from build123d import *

# Parameters (mm, degrees)
F0_R      = 50
F1_DEPTH  = 60
F3_DEPTH  = 60.001
F4_W      = 50
F4_H      = 50
F5_DEPTH  = 140
F6_W      = 30
F6_H      = 59.9
F7_DEPTH  = 49.99
F13_DEPTH = 50.0010001
F15_DEPTH = 50.0010001


with BuildPart() as f1:
    # F0 (on Top) → F1 (new body)
    with BuildSketch(Plane.XY):
        Circle(F0_R)
    extrude(amount=F1_DEPTH)

    # F2 (on face) → F3 (cut, through all)
    with BuildSketch(Plane.XY.offset(60)):
        with BuildLine():
            Line((0, -50), (0, 0))
            Line((0, 0), (-50, 0))
            ThreePointArc((-50, 0), (-35.3553390593, -35.3553390593), (0, -50))
        make_face()
    extrude(amount=-F3_DEPTH, mode=Mode.SUBTRACT)

    # F4 (on Top) → F5 (join)
    with BuildSketch(Plane.XY):
        with Locations((-25, -25)):
            Rectangle(F4_W, F4_H)
    extrude(amount=F5_DEPTH)

    # F6 (on face) → F7 (cut)
    with BuildSketch(Plane(origin=(-50, 0, 0), x_dir=(0, -1, 0), z_dir=(-1, 0, 0))):
        with Locations((35, 29.95)):
            Rectangle(F6_W, F6_H)
    extrude(amount=-F7_DEPTH, mode=Mode.SUBTRACT)

    # F5_face2 (on face) → F9 section 0
    with BuildSketch(Plane(origin=(-24.9962622307, -50, 99.9395321524), x_dir=(1, 0, 0), z_dir=(0, -1, 0)), mode=Mode.PRIVATE) as f9_s0:
        Polygon((-25.0037377693, -40.0395321524), (24.9862622307, -40.0395321524), (24.9862622307, -99.9395321524), (24.9962622307, -99.9395321524), (24.9962622307, -39.9395321524), (24.9962622307, 40.0604678476), (-25.0037377693, 40.0604678476), align=None)
    loft([f9_s0.sketch, Vertex(-50, -20, 140)], mode=Mode.SUBTRACT)

    # F10 (on face) → F11 section 0
    with BuildSketch(Plane.XY.offset(140), mode=Mode.PRIVATE) as f11_s0:
        Polygon((-50, 0), (-50, -20), (0, 0), align=None)
    loft([f11_s0.sketch, Vertex(0, 0, 60)], mode=Mode.SUBTRACT)

    # F12 (on Front) → F13 (cut, through all)
    with BuildSketch(Plane.XZ):
        Polygon((50, 60.5232338582), (0, 60.5232338582), (50, 30.5232338582), align=None)
    extrude(amount=F13_DEPTH, mode=Mode.SUBTRACT)

    # F14 (on Right) → F15 (cut, through all)
    with BuildSketch(Plane.YZ):
        with BuildLine():
            Line((0, 29.99), (0, 0))
            Line((0, 0), (50, 0))
            ThreePointArc((50, 0), (28.8876713773, 21.4766128331), (0, 29.99))
        make_face()
    extrude(amount=F15_DEPTH, mode=Mode.SUBTRACT)


solid = f1.part
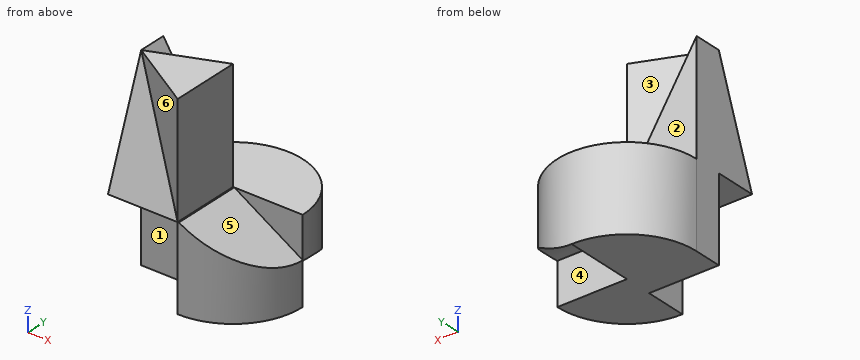
Design review of the part built by this model. Coordinates are the model's own, in mm. Face numbers are marked on the shaded views. A direction names the side the tool comes from. Round coordinates to 2 decimals unless told otherwise and drop trailing zeros. Loops run counter-clockwise (first coordinate to the right, second up) from the corner with the lowest first, then second, coordinate; pieces in that order, holes last. Notation, with made-up numbers: (89.25, -2) - (130.25, -2) arc R13 ccw to (130.25, 9) - close; hole circle Ø6 at (46, 56.5). An arc over 180 degrees is marked (long way). One line per item, written item: value. Start each with the question number.
1) Draft analysis for pull direction X (two halves, no side actions). For the marked faces 4, 5 and 6, state which applies: +X half, -X half, draft (parallel to the pull), parting line (faces both ways), or undercut.
2) Consider section B-B on z = 69. Give the boundary of the cut face in (x, y) (3 decimals), then the cut area to 3 significant figures.
3) For the marked faces 1, 2 and 3, list the 3-axis set-ups (+Z, -Z, +X, -X, +Y, -Y) from which the entire face can be reached by the end or side of a thin tool; tool diameter is ignored.
4) Consider section A-A on x = -14.5. Give the boundary of the cut face in (y, z), then the cut area to 3 significant figures.
5) Insertion check: pin 1 Ø9 at (x, y) = (-14.5, -29.5) entering from -Z; pin 2 Ø3 at (x, z) = (-3.5, 35.5) entering from +Y; pin 3 Ø24 at (x, z) = (34.5, 10.5) entering from +Y. Each pin has a flat end and moves straight along its axis. Give the tip position at first contact, or say it passes through.
6) Consider section D-D on y = 38.5. Give the boundary of the cut face in (x, z).
7) To check wall thickness, follow L1, parallel to Z at x = -25, y = 2; L2, parallel to X at y = -31.5, z = 80; L3, parallel to Z at x = 25, y = 1.5. State the ranges of each line that lie inside material, in increasing order. Write a range as from..to.
Reported:
1. face 4: draft
1. face 5: +X half
1. face 6: undercut
2. outline: (-50, -46.592) - (-5.689, -46.592) - (-24.648, -35.214) - (-24.643, -35.214) - (0, -50) - (0, 0) - (-5.625, -2.25) - (-5.625, 0) - (-50, 0) - close
2. area: 2,330 mm^2
3. face 1: -Z, -X, -Y
3. face 2: +Z, +X, -X, +Y
3. face 3: +Z, +Y
4. outline: (-50, 59.9) - (-41.3, 59.9) - (-41.3, 83.12) - close; (-41.3, 59.9) - (-20, 59.9) - (-20, 0) - (47.85, 0) - (47.85, 60) - (0, 60) - (0, 83.2) - (-5.8, 83.2) - (-5.8, 140) - (-41.3, 140) - close
4. area: 7,150 mm^2
5. pin 1: stops at z = 59.9
5. pin 2: stops at y = 49.96
5. pin 3: stops at y = 44.65
6. outline: (-31.9, 0) - (0, 0) - (0, 14.31) - (31.9, 14.31) - (31.9, 60) - (-31.9, 60) - close
7. L1: z = 0..60
7. L2: x = -50..0
7. L3: z = 29.92..60
